```python
from build123d import *

# Parameters (mm, degrees)
F0_W     = 139.7
F0_H     = 73.025
F1_DEPTH = 19.05
F2_W     = 25.4
F2_H     = 12.7
F2_R     = 6.35
F3_DEPTH = 25.4
F5_D     = 5.1054
F5_DEPTH = 16.51
F5_TIP   = 1.5338169022


with BuildPart() as f1:
    # F0 (on Top) → F1 (new body)
    with BuildSketch(Plane.XY):
        with Locations((69.85, 36.5125)):
            Rectangle(F0_W, F0_H)
    extrude(amount=F1_DEPTH)

    # F2 (on face) → F3 (cut)
    with BuildSketch(Plane.XY.offset(19.05)):
        with Locations((12.7, 28.575)):
            Rectangle(F2_W, F2_H)
        with Locations((101.6, 28.575)):
            Circle(F2_R)
    extrude(amount=-F3_DEPTH, mode=Mode.SUBTRACT)

    # F5
    with Locations(Plane.XY.offset(19.05)):
        with Locations((18.6944, 52.07), (118.11, 52.07)):
            Hole(F5_D / 2, depth=F5_DEPTH)
            with Locations((0, 0, -(F5_DEPTH + F5_TIP / 2))):  # 118° drill point
                Cone(0, F5_D / 2, F5_TIP, mode=Mode.SUBTRACT)


solid = f1.part
```
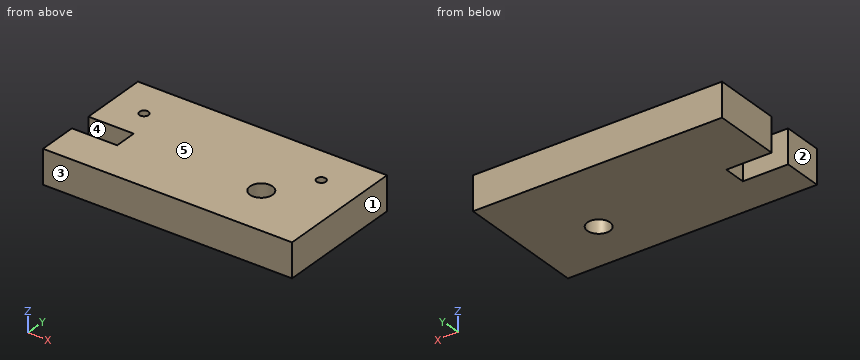
Check sheet for the modelled part. Datum: model origin and axes. Units: mm. Face numbers are marked on the shaded views. A direction names the side the tool comes from. Give positions to 0.01 mm unless a question says otherwise; leave off trailing zeros. Order: outer loops, then holes, each group sorted by start corner. A loop starts at its lowest first (then second) coordinate and runs counter-clockwise, first axis right, second up. Notation, with made-up numbers: M 60.25,10 L 108.25,10 A20 ccw 108.25,25 Z; hole C -10,49 d4. An arc over 180 degrees is marked long. Answer in a Markdown table with one row per item. Add a question column.
Q1. Sectioned sample at A-A, the plane x = 101.6. Record the boundary of the cut face in (y, z) (3 decimals).
Q2. Release check for a two-part mould opening along X. For the marked faces 1, 2 and 3 record: released by +X, released by -X, zero draft, split by the parting line, or undercut.
Q3. Access from +Z, -Z, +X, -X, +Y, -Y to the whole of each face (thin tool, end or side, straight path). Record for the marked faces 4 and 5.
Q4. Gauge pin test, flat end, axial feed: pin 1 Ø16.5 at (x, y) = (101.6, 28.575) entering from +Z. Record the tip position at first contact, or that the pin passes through.
Q5. Sectioned sample at B-B, the plane z = 10.5. Record the boundary of the cut face in (x, y) (3 decimals), and give its area (3 significant figures).
Q6. Thickness scan on L1, parallel to X at y = 52.07, z = 15.75; L2, parallel to Y at x = 13, z = 15.25 (3 decimals); L3, parallel to Y at x = 118.11, z = 15.5 (3 decimals). Record the ranges inside material, lowest first.
Verdict:
| question | item | result |
|---|---|---|
| 1 | outline | M 0,0 L 22.225,0 L 22.225,19.05 L 0,19.05 Z; M 34.925,0 L 73.025,0 L 73.025,19.05 L 34.925,19.05 Z |
| 2 | face 1 | released by +X |
| 2 | face 2 | released by -X |
| 2 | face 3 | zero draft |
| 3 | face 4 | +Z, -Z, -X |
| 3 | face 5 | +Z, +X, -X, +Y, -Y |
| 4 | pin 1 | z = 19.05 |
| 5 | outline | M 0,0 L 139.7,0 L 139.7,73.025 L 0,73.025 L 0,34.925 L 25.4,34.925 L 25.4,22.225 L 0,22.225 Z; hole C 18.694,52.07 d5.105; hole C 101.6,28.575 d12.7; hole C 118.11,52.07 d5.105 |
| 5 | area | 9,710 mm² |
| 6 | L1 | 0 to 16.14, 21.25 to 115.56, 120.66 to 139.7 |
| 6 | L2 | 0 to 22.225, 34.925 to 73.025 |
| 6 | L3 | 0 to 49.517, 54.623 to 73.025 |
